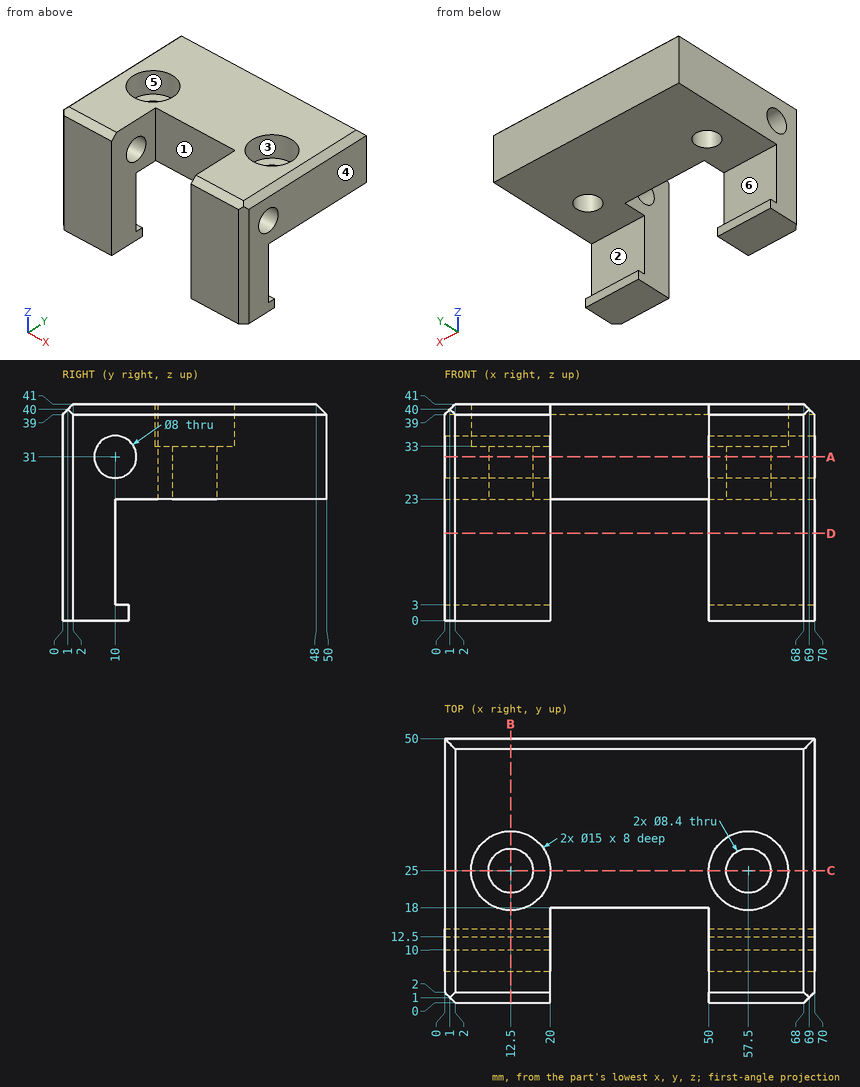
Could you check a few things on this drawing? It's one solid part, dimensions in mm from its lowest x, y, z. A direction names the side the tool comes from. Coordinates: 2 decimals unless noted, no trailing zeros. Order: outer loops, then holes, each group sorted by start corner. A loop starts at its lowest first (then second) coordinate and runs counter-clockwise, first axis right, second up. Notation, with made-up numbers: (26.25, 60) -> (41.25, 60) arc R33 cw to (41.25, 92) -> close; hole circle Ø3 at (47, -11). An arc over 180 degrees is marked (long way). One line per item, written item: value. Start each with the question number.
1) We'd pull the mould along X, two halves only. Please class the marked faces 4, 5 and 6: +X half, -X half, draft (parallel to the pull), parting line (faces both ways), or undercut.
2) Imagine slicing it at D-D on z = 16.5. List the corners of the cut face in (x, y) for me.
3) Imagine slicing it at B-B on x = 12.5. List the corners of the cut face in (y, z) for me.
4) If I drill on L1, parallel to X at y = 25, z = 35.5; L2, parallel to X at y = 25, z = 28.5; L3, parallel to Y at x = 12.5, z = 37.5, over which ranges is the centre line in solid material (lowest first)? Write a range as [from, to].
5) Imagine slicing it at A-A on z = 31. List the corners of the cut face in (x, y) for me, plus the area to 3 significant figures.
6) Which directions (+Z, -Z, +X, -X, +Y, -Y) give clear straight access to the entire face, cutting with the end or side of a thin tool? Please do the marked faces 1, 2 and 3.
7) Imagine slicing it at C-C on y = 25. List the corners of the cut face in (x, z) for me.
8) I'm going to push flat-ended pins straight in: pin 1 (6.5 mm diameter, centred on y = 10, z = 31, fed in from +X); pin 2 (3.5 mm diameter, centred on x = 63, z = 2, fed in from +Y); pin 3 (2 mm diameter, centred on x = 15.5, y = 20, fed in from -Z); pin 4 (9 mm diameter, centred on x = 37, z = 29, fed in from -Y). Where does each tip first touch, or does it pass through?
Answer list:
1. face 4: +X half
1. face 5: undercut
1. face 6: draft
2. outline: (0, 2) -> (2, 0) -> (20, 0) -> (20, 10) -> (0, 10) -> close; (50, 0) -> (68, 0) -> (70, 2) -> (70, 10) -> (50, 10) -> close
3. outline: (0, 0) -> (12.5, 0) -> (12.5, 3) -> (10, 3) -> (10, 23) -> (20.8, 23) -> (20.8, 33) -> (17.5, 33) -> (17.5, 41) -> (2, 41) -> (0, 39) -> close; (29.2, 23) -> (50, 23) -> (50, 39) -> (48, 41) -> (32.5, 41) -> (32.5, 33) -> (29.2, 33) -> close; hole circle Ø8 at (10, 31)
4. L1: x = [0, 5], [20, 50], [65, 70]
4. L2: x = [0, 8.3], [16.7, 53.3], [61.7, 70]
4. L3: y = [0, 17.5], [32.5, 50]
5. outline: (0, 2) -> (2, 0) -> (20, 0) -> (20, 6) -> (0, 6) -> close; (0, 14) -> (20, 14) -> (20, 18) -> (50, 18) -> (50, 14) -> (70, 14) -> (70, 50) -> (0, 50) -> close; (50, 0) -> (68, 0) -> (70, 2) -> (70, 6) -> (50, 6) -> close; hole circle Ø8.4 at (12.5, 25); hole circle Ø8.4 at (57.5, 25)
5. area: 2,530 mm2
6. face 1: +Z, -Z, -Y
6. face 2: +X, -X, +Y
6. face 3: +Z
7. outline: (0, 23) -> (8.3, 23) -> (8.3, 33) -> (5, 33) -> (5, 41) -> (2, 41) -> (0, 39) -> close; (16.7, 23) -> (53.3, 23) -> (53.3, 33) -> (50, 33) -> (50, 41) -> (20, 41) -> (20, 33) -> (16.7, 33) -> close; (61.7, 23) -> (70, 23) -> (70, 39) -> (68, 41) -> (65, 41) -> (65, 33) -> (61.7, 33) -> close
8. pin 1: passes through
8. pin 2: stops at y = 12.5
8. pin 3: stops at z = 23
8. pin 4: stops at y = 18
